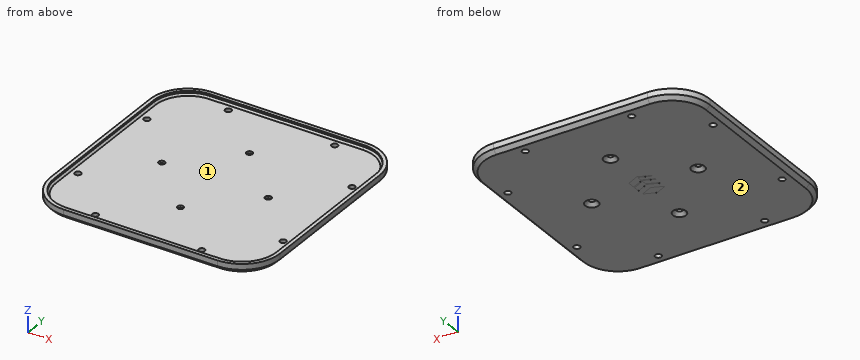
Autodesk Inventor part; units mm, degrees
ref_plane "YZ Plane" through (0, 0, 0) normal (1, 0, 0) x (0, 1, 0)
ref_plane "XZ Plane" through (0, 0, 0) normal (0, 1, 0) x (-1, 0, 0)
ref_plane "XY Plane" through (0, 0, 0) normal (0, 0, 1) x (1, 0, 0)
sketch "Sketch1" plane through (0, 0, 0) normal (0, 0, 1) x (1, 0, 0)
  line L0 (20, 0) -> (101, 0)
  line L1 (121, 20) -> (121, 101)
  line L2 (101, 121) -> (20, 121)
  line L3 (0, 101) -> (0, 20)
  arc A0 (20, 121) -> (0, 101) centre (20, 101) ccw
  arc A1 (121, 101) -> (101, 121) centre (101, 101) ccw
  arc A2 (101, 0) -> (121, 20) centre (101, 20) ccw
  arc A3 (0, 20) -> (20, 0) centre (20, 20) ccw
  point P0 (0, 0)
  point P1 (121, 121)
  point P2 (121, 0)
  point P3 (0, 121)
  dimension "d0" = 121
  dimension "d1" = 121
  dimension "d2" = 20
extrude "Extrusion1" add sketch "Sketch1" along normal blind 3
sketch "Sketch2" plane through (0, 0, 3) normal (0, 0, 1) x (1, 0, 0)
  arc A0 (101, 0) -> (121, 20) centre (101, 20) ccw
  line L0 (121, 20) -> (121, 101)
  arc A1 (121, 101) -> (101, 121) centre (101, 101) ccw
  line L1 (101, 121) -> (20, 121)
  arc A2 (20, 121) -> (0, 101) centre (20, 101) ccw
  line L2 (0, 101) -> (0, 20)
  arc A3 (0, 20) -> (20, 0) centre (20, 20) ccw
  line L3 (20, 0) -> (101, 0)
  line L4 (20, 119.05) -> (101, 119.05)
  arc A4 (119.05, 101) -> (101, 119.05) centre (101, 101) ccw
  line L5 (119.05, 101) -> (119.05, 20)
  arc A5 (101, 1.95) -> (119.05, 20) centre (101, 20) ccw
  line L6 (101, 1.95) -> (20, 1.95)
  arc A6 (1.95, 20) -> (20, 1.95) centre (20, 20) ccw
  line L7 (1.95, 20) -> (1.95, 101)
  arc A7 (20, 119.05) -> (1.95, 101) centre (20, 101) ccw
  point P0 (0, 0)
  dimension "d5" = 1.95
extrude "Extrusion2" add sketch "Sketch2" along normal blind 2
chamfer "Chamfer1" distance 1 angle 45 8 edges at (1.95, 60.5, 3) (7.2367, 7.2367, 3) (60.5, 1.95, 3) (113.7633, 7.2367, 3) (119.05, 60.5, 3) (113.7633, 113.7633, 3) (60.5, 119.05, 3) (7.2367, 113.7633, 3)
sketch "Sketch3" plane through (0, 0, 0) normal (0, 0, -1) x (-1, 0, 0)
  circle A0 centre (-6.5, 88.5) radius 2.15
  circle A1 centre (-6.5, 32.5) radius 2.15
  circle A2 centre (-32.5, 6.5) radius 2.15
  circle A3 centre (-88.5, 6.5) radius 2.15
  circle A4 centre (-114.5, 32.5) radius 2.15
  circle A5 centre (-114.5, 88.5) radius 2.15
  circle A6 centre (-88.5, 114.5) radius 2.15
  circle A7 centre (-32.5, 114.5) radius 2.15
  circle A8 centre (-60.5, 60.5) radius 2.15
  circle A9 centre (-60.5, 88.5) radius 2.15
  circle A10 centre (-88.5, 60.5) radius 2.15
  circle A11 centre (-60.5, 32.5) radius 2.15
  circle A12 centre (-32.5, 60.5) radius 2.15
  circle A13 centre (-88.5, 114.5) radius 1.65
  circle A14 centre (-32.5, 114.5) radius 1.65
  circle A15 centre (-60.5, 88.5) radius 1.65
  circle A16 centre (-114.5, 88.5) radius 1.65
  circle A17 centre (-88.5, 60.5) radius 1.65
  circle A18 centre (-60.5, 60.5) radius 1.65
  circle A19 centre (-32.5, 60.5) radius 1.65
  circle A20 centre (-6.5, 88.5) radius 1.65
  circle A21 centre (-6.5, 32.5) radius 1.65
  circle A22 centre (-60.5, 32.5) radius 1.65
  circle A23 centre (-114.5, 32.5) radius 1.65
  circle A24 centre (-88.5, 6.5) radius 1.65
  circle A25 centre (-32.5, 6.5) radius 1.65
  point P0 (0, 0)
  dimension "d11" = 3.3
  dimension "d12" = 3.3
  dimension "d13" = 3.3
  dimension "d14" = 3.3
  dimension "d15" = 3.3
  dimension "d16" = 3.3
  dimension "d17" = 3.3
  dimension "d18" = 3.3
  dimension "d19" = 3.3
  dimension "d20" = 3.3
  dimension "d21" = 3.3
  dimension "d22" = 3.3
  dimension "d23" = 3.3
extrude "Extrusion3" cut sketch "Sketch3" against normal through all contours A13 | A14 | A15 | A16 | A17 | A19 | A20 | A21 | A22 | A23 | A24 | A25
chamfer "Chamfer2" distance 1.8 angle 45 4 edges at (62.15, 88.5, 0) (90.15, 60.5, 0) (34.15, 60.5, 0) (62.15, 32.5, 0)
chamfer "Chamfer3" distance 2 angle 45 8 edges at (60.5, 121, 0) (5.8579, 115.1421, 0) (0, 60.5, 0) (5.8579, 5.8579, 0) (60.5, 0, 0) (115.1421, 5.8579, 0) (121, 60.5, 0) (115.1421, 115.1421, 0)
sketch "Sketch4" plane through (0, 0, 0) normal (0, 0, -1) x (-1, 0, 0)
  line L0 (-53.168, 55.5218) -> (-59.1357, 52.7365)
  line L1 (-59.1357, 52.7365) -> (-65.1751, 55.2519)
  line L2 (-65.1751, 55.2519) -> (-59.2074, 58.0372)
  line L3 (-59.2074, 58.0372) -> (-53.168, 55.5218)
  line L4 (-53.168, 59.4718) -> (-59.2074, 61.9872)
  line L5 (-59.2074, 61.9872) -> (-59.2074, 64.5372)
  line L6 (-59.2074, 64.5372) -> (-65.1751, 61.7519)
  line L7 (-65.1751, 61.7519) -> (-65.1751, 58.5019)
  line L8 (-53.168, 59.4718) -> (-53.168, 58.7718)
  line L9 (-53.168, 58.7718) -> (-59.2074, 61.2872)
  line L10 (-59.2074, 61.2872) -> (-65.1751, 58.5019)
  line L11 (-59.2074, 69.1872) -> (-65.1751, 66.359)
  line L12 (-59.2074, 65.9372) -> (-59.2074, 68.4872)
  line L13 (-53.1419, 63.4218) -> (-59.2074, 65.9372)
  line L14 (-53.1419, 63.4218) -> (-53.1419, 62.7218)
  line L15 (-53.1419, 62.7218) -> (-59.1873, 65.2372)
  line L16 (-65.1751, 66.359) -> (-65.1751, 62.4519)
  line L17 (-59.1873, 65.2372) -> (-65.1751, 62.4519)
  line L18 (-59.2074, 69.1872) -> (-53.1419, 66.6718)
  line L19 (-53.1419, 66.6718) -> (-53.1419, 65.9718)
  line L20 (-53.1419, 65.9718) -> (-59.2074, 68.4872)
  point P0 (0, 0)
  dimension "d32" = 0.7
  dimension "d33" = 0.7
  dimension "d34" = 0.7
  dimension "d35" = 0.7
  dimension "d36" = 0
  dimension "d37" = 3.25
  dimension "d38" = 0.7
  dimension "d39" = 0.7
  dimension "d40" = 0.7
  dimension "d41" = 0.7
  dimension "d42" = 3.25
  dimension "d43" = 3.25
  dimension "d44" = 3.25
  dimension "d45" = 3.25
  dimension "d46" = 3.25
  dimension "d47" = 3.25
extrude "Extrusion4" cut sketch "Sketch4" against normal blind 0.01
equation "\"d12\" = d11"
equation "\"d13\" = d11"
equation "\"d14\" = d11"
equation "\"d15\" = d11"
equation "\"d16\" = d11"
equation "\"d17\" = d11"
equation "\"d18\" = d11"
equation "\"d19\" = d11"
equation "\"d20\" = d11"
equation "\"d21\" = d20"
equation "\"d22\" = d20"
equation "\"d23\" = d20"
equation "\"d33\" = d32"
equation "\"d34\" = d32"
equation "\"d38\" = d32"
equation "\"d39\" = d32"
equation "\"d40\" = d32"
equation "\"d41\" = d32"
equation "\"d42\" = d37"
equation "\"d44\" = d42"
equation "\"d45\" = d44"
equation "\"d46\" = d45"
equation "\"d47\" = d45"
properties part number "battery_pack_cover_rear" material "ABS Plastic"
Part model, mm, in its own coordinate system. Face numbers are marked on the shaded views. Round coordinates to 2 decimals unless told otherwise and drop trailing zeros. Order: outer loops, then holes, each group sorted by start corner. A loop starts at its lowest first (then second) coordinate and runs counter-clockwise, first axis right, second up. Notation, with made-up numbers: M -37,-7 L 19,-7 A12 cw 19,-1 Z; hole C -21.75,-19.75 d1. An arc over 180 degrees is marked long. Put each result on its own line as item: value. Start each with the question number.
1. Drop flat-ended pins along their axis: pin 1 (2 mm diameter, centred on x = 32.5, y = 6.5, fed in from +Z); pin 2 (5.5 mm diameter, centred on x = 114.5, y = 32.5, fed in from -Z); pin 3 (2 mm diameter, centred on x = 16.5, y = 15.5, fed in from +Z). Give the stop position or say it passes through.
2. Drill centre lines: probe 1 along Y at (x, z) = (60.5, 2.75); probe 2 along Y at (x, z) = (32.5, 2.15); probe 3 along X at (y, z) = (42.5, 4.2). Where is each one in solid material? Low to high. Write a range as [from, to].
3. Slice it at A-A on x = 88.5. List the corners of the cut face in (y, z), then the cut area to 3 significant figures.
4. Two-plate mould, pull along Y, no slides. Class the marked faces 1 and 2: +Y half, -Y half, draft (parallel to the pull), parting line (faces both ways), or undercut.
Findings:
1. pin 1: through
1. pin 2: z = 0
1. pin 3: z = 3
2. probe 1: [0, 30.85], [34.15, 86.85], [90.15, 121]
2. probe 2: [0, 4.85], [8.15, 58.85], [62.15, 112.85], [116.15, 121]
2. probe 3: [0, 1.95], [119.05, 121]
3. outline: M 0,2 L 2,0 L 4.85,0 L 4.85,3 L 2.95,3 L 1.95,4 L 1.95,5 L 0,5 Z; M 8.15,0 L 57.05,0 L 58.85,1.8 L 58.85,3 L 8.15,3 Z; M 62.15,1.8 L 63.95,0 L 112.85,0 L 112.85,3 L 62.15,3 Z; M 116.15,0 L 119,0 L 121,2 L 121,5 L 119.05,5 L 119.05,4 L 118.05,3 L 116.15,3 Z
3. area: 335 mm2
4. face 1: undercut
4. face 2: draft
